For this review, take the finished solid that the model builds, in its own axes (mm). Face numbers are marked on the shaded views. A direction names the side the tool comes from. Coordinates: 2 decimals unless noted, no trailing zeros. Write each loop counter-clockwise with the first axis right and the second up, starting at its lowest first coordinate (ties: lowest second). Pieces come first, ordered by that corner, then holes. Notation, with made-up numbers: (-30, 70.5) -> (27, 70.5) arc R19 ccw to (27, 102.5) -> close; hole circle Ø2 at (-6.5, 78.5). An arc over 180 degrees is marked (long way). Put each result on its own line as item: value. Start each with the question number.
Item 1: Consider section A-A on x = 3. Give the boundary of the cut face in (y, z), and give its area (3 significant figures).
Item 2: Consider section C-C on y = -1.75. Give the boundary of the cut face in (x, z).
Item 3: Consider section B-B on z = -3. Give the boundary of the cut face in (x, y).
Item 4: The part is to be moulded in two halves that separate along Z. For the marked faces 3, 4, 5 and 6, say which applies: +Z half, -Z half, draft (parallel to the pull), parting line (faces both ways), or undercut.
Item 5: Consider section D-D on x = 5.3. Give the boundary of the cut face in (y, z).
Item 6: To check wall thickness, follow L1, parallel to Z at x = 1.95, y = 3; L2, parallel to Z at x = 3, y = -2; L3, parallel to Y at x = 1.95, z = -3. State the ranges of each line that lie inside material, in increasing order.
Item 7: Insertion check: P1, Ø1.2, axis at x = 3, z = -2.5, coming from the -Y side. The pin has a flat end and moves straight along its axis. Give the tip position at first contact, or say it passes through.
Item 8: For the marked faces 1 and 2, list the 3-axis set-ups (+Z, -Z, +X, -X, +Y, -Y) from which the entire face can be reached by the end or side of a thin tool; tool diameter is ignored.
Autodesk Inventor part; units mm, degrees
ref_plane "YZ Plane" through (0, 0, 0) normal (1, 0, 0) x (0, 1, 0)
ref_plane "XZ Plane" through (0, 0, 0) normal (0, 1, 0) x (-1, 0, 0)
ref_plane "XY Plane" through (0, 0, 0) normal (0, 0, 1) x (1, 0, 0)
sketch "Esboço1" plane through (0, 0, 0) normal (1, 0, 0) x (0, 1, 0)
  line L0 (0, 0) -> (6, 0)
  line L1 (6, 0) -> (6, -6)
  line L2 (6, -6) -> (0, -6)
  line L3 (0, -6) -> (0, 0)
  dimension "d0" = 6
  dimension "d1" = 6
extrude "Extrusão1" add sketch "Esboço1" along normal blind 6
sketch "Esboço2" plane through (0, 0, 0) normal (0, 0, 1) x (1, 0, 0)
  point P0 (0, 0)
sketch "Esboço3" plane through (6, 0, 0) normal (1, 0, 0) x (0, 0, -1)
  line L0 (0, 6) -> (0, 0)
  line L1 (6, 0) -> (6, 6)
sketch "Esboço4" plane through (0, 0, -6) normal (0, -1, 0) x (1, 0, 0)
  line L0 (0, 0) -> (0, 6)
  line L1 (6, 0) -> (6, 6)
  circle A0 centre (3, 3) radius 2
  dimension "d5" = 4
extrude "Extrusão2" add sketch "Esboço4" along normal blind 2.5
sketch "Esboço6" plane through (0, 0, 0) normal (-1, 0, 0) x (0, 0, 1)
  line L0 (-6, 6) -> (0, 6)
  line L1 (0, 0) -> (-6, 0)
  point P0 (-3, 3)
hole "Furo2" at (0, 3, -3) direction (1, 0, 0) diameter 3.242 depth 4
fillet "Arredondamento1" radius 1 1 edges at (6, 3, 0)
fillet "Arredondamento2" radius 1 3 edges at (6, 6, -3.5) (5.7071, 6, -0.2929) (2.5, 6, 0)
fillet "Arredondamento3" radius 1 3 edges at (0, 6, -3.5) (0, 5.7071, -0.2929) (0, 2.5, 0)
fillet "Arredondamento4" radius 1 5 edges at (0, 2.5, -6) (0.2929, 5.7071, -6) (3, 6, -6) (5.7071, 5.7071, -6) (6, 2.5, -6)
sketch "Esboço7" plane through (3, -2.5, -3) normal (0, -1, 0) x (1, 0, 0)
  point P0 (-3, 3)
sketch "Esboço8" plane through (3, -2.5, -3) normal (0, -1, 0) x (1, 0, 0)
  point P0 (-3, 3)
  point P1 (0, 0)
hole "Furo3" at (3, -2.5, -3) direction (0, 1, 0) diameter 2.459 depth 2
properties part number "CONECTOR R-F"
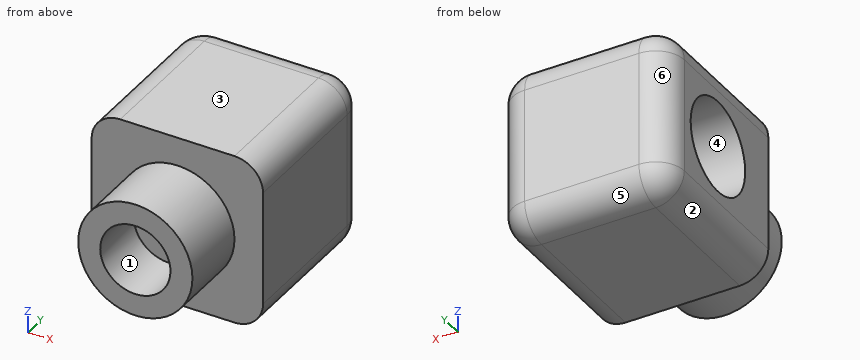
Return value:
1. outline: (-2.5, -5) -> (0, -5) -> (0, -6) -> (5, -6) arc R1 ccw to (6, -5) -> (6, -1) arc R1 ccw to (5, 0) -> (0, 0) -> (0, -1) -> (-2.5, -1) -> (-2.5, -1.77) -> (-0.5, -1.77) -> (-0.5, -4.23) -> (-2.5, -4.23) -> close; hole circle Ø3.24 at (3, -3)
1. area: 32.4 mm^2
2. outline: circle Ø4 at (3, -3); hole circle Ø2.46 at (3, -3)
3. outline: (0, 0) -> (1, 0) -> (1, -2.5) -> (1.77, -2.5) -> (1.77, -0.5) -> (4.23, -0.5) -> (4.23, -2.5) -> (5, -2.5) -> (5, 0) -> (6, 0) -> (6, 5) arc R1 ccw to (5, 6) -> (1, 6) arc R1 ccw to (0, 5) -> (0, 4.62) -> (4, 4.62) -> (4, 1.38) -> (0, 1.38) -> close
4. face 3: +Z half
4. face 4: undercut
4. face 5: -Z half
4. face 6: draft
5. outline: (0, -5.95) -> (5, -5.95) arc R0.95 ccw to (5.95, -5) -> (5.95, -1) arc R0.95 ccw to (5, -0.05) -> (0, -0.05) -> close
6. L1: -6 to -4.62, -1.38 to 0
6. L2: -5 to -4.23, -1.77 to -1
6. L3: -0.5 to 1.38, 4.62 to 6
7. P1: y = -0.5
8. face 1: -Y
8. face 2: -Z, -X, +Y, -Y
